Part model, mm, in its own coordinate system. A direction names the side the tool comes from. Give positions to 0.01 mm unless a question says otherwise; leave off trailing zeros. Order: outer loops, then holes, each group sorted by start corner. A loop starts at its lowest first (then second) coordinate and runs counter-clockwise, first axis right, second up. Notation, with made-up numbers: (26, -20) -> (33, -20) arc R28 ccw to (33, 15) -> close; hole circle Ø8 at (-27.5, 58.5). An arc over 180 degrees is marked (long way). Write item = value, one per line. Start each with the question number.
(1) Saw through at D-D, the plane x = 4. List the corners of the cut face in (y, z).
(2) Saw through at B-B, the plane y = -62.5. List the corners of the cut face in (x, z), then the cut area to 3 significant figures.
(3) Probe line 1 along Y through (x, z) = (9.5, 13.1); line 2 along X through (y, z) = (-62, 11.5); line 3 along X through (y, z) = (-64, 12.1). List the from-to ranges inside material, lowest first. Write a range as from..to.
(4) Two-plate mould, pull along X, no slides. Class faces 1 (the flat face through (6.445, -63.904, 12.482)), 2 (the flat face through (6.73, -62.16, 12.48)), 3 (the flat face through (3.66, -63.97, 12.48)), 4 (the flat face through (6.5, -61.149, 12.5)): pulls with the +X half, pulls with the -X half, needs draft (parallel to the pull), parting line crosses it, or undercut.
(5) Saw through at C-C, the plane x = 6.5. List the corners of the cut face in (y, z), then the cut area to 3 significant figures.
(6) Saw through at A-A, the plane z = 13.4. List the corners of the cut face in (x, y), then the cut area to 3 significant figures.
(7) Which spindle directions (+Z, -Z, +X, -X, +Y, -Y) get a long thin tool onto all of the face, cutting with end or side? Do faces 5 (the flat face through (6.244, -70.563, 12.482)), 6 (the flat face through (4.2, -62.91, 12.48)). Say none if no direction does.
(8) Flat gauge pins, fed straight in: pin 1 (1 mm diameter, centred on x = 4, z = 12.5, fed in from +Y); pin 2 (1 mm diameter, centred on y = -68, z = 12.5, fed in from -X). Where does each tip first touch, or does it go through?
from build123d import *

# Parameters (mm, degrees)
MAIN_EXTRUDE_DEPTH    = 25
BOTTOM_FOOT_CUT_DEPTH = 26
TALON_CUTS_DEPTH      = 26
ANKLE_FILLETS_R       = 10
INNER_LEG_FILLET_R    = 20
KNEE_FILLET_R         = 20
SCALE1_SCALE          = 0.1
CUT_EXTRUDE3_REACH    = 4.5


with BuildPart() as part:
    # Sketch6 → Main Extrude (new body)
    with BuildSketch(Plane.XY):
        Polygon((0, 0), (-50, 0), (-15, -60), (0, -130), (30, -150), (50, -120), (35, -50), align=None)
    extrude(amount=MAIN_EXTRUDE_DEPTH)

    # Sketch9 → Bottom Foot Cut (cut, through all)
    with BuildSketch(Plane(origin=(0, 0, 0), x_dir=(-1, 0, 0), z_dir=(0, 0, -1))):
        Polygon((-30, -150), (-24.116515946, -146.077677297), (-33.922322703, -144.116515946), align=None)
    extrude(amount=-BOTTOM_FOOT_CUT_DEPTH, mode=Mode.SUBTRACT)

    # Sketch11 → Talon Cuts (cut, through all)
    with BuildSketch(Plane(origin=(0, 0, 0), x_dir=(-1, 0, 0), z_dir=(0, 0, -1))):
        Polygon((-32.941742027, -144.312632081), (-30.980580676, -144.704864351), (-37.869672024, -122.426065595), align=None)
        Polygon((-30.490290338, -144.802922419), (-28.529128986, -145.195154689), (-25.342297799, -124.93154044), align=None)
        Polygon((-28.038838649, -145.293212757), (-26.077677297, -145.685445027), (-13.292661468, -127.341467706), align=None)
    extrude(amount=-TALON_CUTS_DEPTH, mode=Mode.SUBTRACT)

    # Ankle Fillets
    ankle_fillets_edges = [part.edges().sort_by_distance(p)[0] for p in [
        (50, -120, 12.5),
        (0, -130, 12.5),
    ]]
    fillet(ankle_fillets_edges, radius=ANKLE_FILLETS_R)

    # Inner Leg Fillet
    inner_leg_fillet_edges = [part.edges().sort_by_distance(p)[0] for p in [
        (-15, -60, 12.5),
    ]]
    fillet(inner_leg_fillet_edges, radius=INNER_LEG_FILLET_R)

    # Knee Fillet
    knee_fillet_edges = [part.edges().sort_by_distance(p)[0] for p in [
        (35, -50, 12.5),
    ]]
    fillet(knee_fillet_edges, radius=KNEE_FILLET_R)


with BuildPart() as part_1:
    # Scale1: scaled about (7.791739568, -67.94361037, 12.5)
    add(part.part.scale(SCALE1_SCALE).moved(Location((7.012565611, -61.149249333, 11.25))))

    # Sketch12 → Cut-Extrude3 (cut, up to next)
    with BuildSketch(Plane(origin=(0, 0, 11.25), x_dir=(-1, 0, 0), z_dir=(0, 0, -1)), mode=Mode.PRIVATE) as cut_extrude3_sk1:
        Polygon((-6.020782968, -61.149249333), (-7.454438828, -63.197329134), (-5.406359027, -64.630984995), (-2.969144064, -61.149249333), align=None)
    cut_extrude3_tool1 = extrude(cut_extrude3_sk1.sketch, amount=-CUT_EXTRUDE3_REACH, mode=Mode.PRIVATE) & part_1.part
    add(cut_extrude3_tool1.solids().sort_by_distance((5.352502, -62.562677, 11.25))[0], mode=Mode.SUBTRACT)


solid = part_1.part
Results list:
q1.outline = (-64.56, 11.25) -> (-62.62, 11.25) -> (-62.62, 13.75) -> (-64.56, 13.75) -> close
q2.outline = (2.8, 11.25) -> (3.91, 11.25) -> (3.91, 13.75) -> (2.8, 13.75) -> close; (6.97, 11.25) -> (7.96, 11.25) -> (7.96, 13.75) -> (6.97, 13.75) -> close
q2.area = 5.26 mm^2
q3.line_1 = -75.74..-75.55, -75.29..-64.7
q3.line_2 = 2.51..3.56, 6.62..7.61
q3.line_3 = 3.68..4.96, 6.31..9.01
q4.face_1 = undercut
q4.face_2 = undercut
q4.face_3 = pulls with the -X half
q4.face_4 = needs draft
q5.outline = (-71.76, 11.25) -> (-63.87, 11.25) -> (-63.87, 13.75) -> (-71.76, 13.75) -> close; (-61.83, 11.25) -> (-61.15, 11.25) -> (-61.15, 13.75) -> (-61.83, 13.75) -> close
q5.area = 21.4 mm^2
q6.outline = (2.01, -61.15) -> (5.35, -66.87) arc R2 cw to (5.58, -67.46) -> (6.93, -73.75) arc R1 ccw to (7.35, -74.37) -> (9.42, -75.76) -> (9.62, -75.72) -> (8.34, -73.88) -> (9.82, -75.68) -> (9.87, -75.67) -> (9.55, -73.64) -> (10.06, -75.63) -> (10.11, -75.62) -> (10.8, -73.39) -> (10.31, -75.58) -> (10.4, -75.56) -> (11.78, -73.5) arc R1 ccw to (11.92, -72.74) -> (10.6, -66.55) arc R2 ccw to (10.28, -65.82) -> (7.01, -61.15) -> (6.02, -61.15) -> (7.45, -63.2) -> (5.41, -64.63) -> (2.97, -61.15) -> close
q6.area = 62.9 mm^2
q7.face_5 = +Z, -Z, -X, -Y
q7.face_6 = +Z, -Z, +Y
q8.pin_1 = -61.91
q8.pin_2 = 5.59
